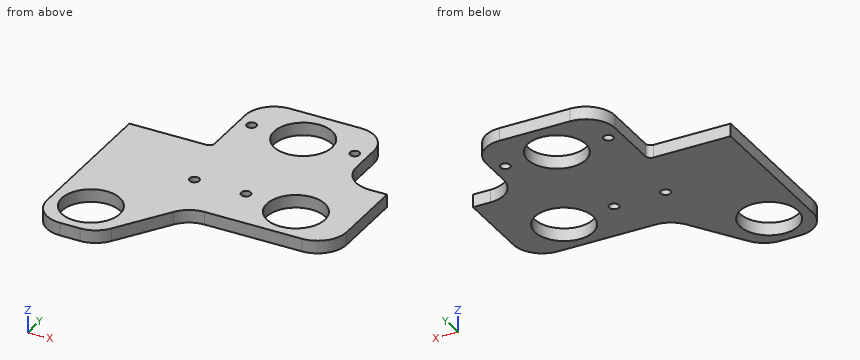
```python
from build123d import *

# Parameters (mm, degrees)
SKETCH1_R           = 14.3129
BOSS_EXTRUDE1_DEPTH = 6.35
FILLET1_R           = 14.2875
SKETCH2_W           = 63.5
SKETCH2_H           = 44.45
BOSS_EXTRUDE2_DEPTH = 6.35
FILLET2_R           = 14.2875
SKETCH3_R           = 14.3129
CUT_EXTRUDE1_DEPTH  = 110.433918417
SKETCH4_R           = 2.38125
SKETCH4_R_2         = 14.2875
CUT_EXTRUDE2_DEPTH  = 110.433918417
SKETCH5_R           = 2.38125
CUT_EXTRUDE3_DEPTH  = 110.433918417
FILLET3_R           = 2.54


with BuildPart() as part:
    # Sketch1 → Boss-Extrude1 (new body)
    with BuildSketch(Plane.XY):
        Polygon((-6.35, -6.35), (63.5, -6.35), (63.5, 44.45), (-63.5, 44.45), (-63.5, -44.45), (-31.75, -44.45), align=None)
        with Locations((-44.45, -25.4)):
            Circle(SKETCH1_R, mode=Mode.SUBTRACT)
        with Locations((35.871852568, 12.7)):
            Circle(SKETCH1_R, mode=Mode.SUBTRACT)
    extrude(amount=BOSS_EXTRUDE1_DEPTH)

    # Fillet1
    fillet1_edges = [part.edges().sort_by_distance(p)[0] for p in [
        (-31.75, -44.45, 3.175),
        (-63.5, -44.45, 3.175),
        (63.5, -6.35, 3.175),
        (-6.35, -6.35, 3.175),
    ]]
    fillet(fillet1_edges, radius=FILLET1_R)

    # Sketch2 → Boss-Extrude2 (add)
    with BuildSketch(Plane.XY.offset(6.35)):
        with Locations((8.89, 66.675)):
            Rectangle(SKETCH2_W, SKETCH2_H)
    extrude(amount=-BOSS_EXTRUDE2_DEPTH)

    # Fillet2
    fillet2_edges = [part.edges().sort_by_distance(p)[0] for p in [
        (-22.86, 88.9, 3.175),
        (40.64, 88.9, 3.175),
        (40.64, 44.45, 3.175),
    ]]
    fillet(fillet2_edges, radius=FILLET2_R)

    # Sketch3 → Cut-Extrude1 (cut, through all)
    with BuildSketch(Plane.XY.offset(6.35)):
        with Locations((9.062967637, 68.577618639)):
            Circle(SKETCH3_R)
    extrude(amount=-CUT_EXTRUDE1_DEPTH, mode=Mode.SUBTRACT)

    # Sketch4 → Cut-Extrude2 (cut, through all)
    with BuildSketch(Plane.XY.offset(6.35)):
        with Locations((-16.337032363, 68.577618639)):
            Circle(SKETCH4_R)
        with Locations((34.462967637, 68.577618639)):
            Circle(SKETCH4_R)
        with Locations((9.062967637, 68.577618639)):
            Circle(SKETCH4_R_2)
    extrude(amount=-CUT_EXTRUDE2_DEPTH, mode=Mode.SUBTRACT)

    # Sketch5 → Cut-Extrude3 (cut, through all)
    with BuildSketch(Plane.XY.offset(6.35)):
        with Locations((-15.875, 15.875)):
            Circle(SKETCH5_R)
        with Locations((9.525, 15.875)):
            Circle(SKETCH5_R)
    extrude(amount=-CUT_EXTRUDE3_DEPTH, mode=Mode.SUBTRACT)

    # Fillet3
    fillet3_edges = [part.edges().sort_by_distance(p)[0] for p in [
        (-22.86, 44.45, 3.175),
    ]]
    fillet(fillet3_edges, radius=FILLET3_R)


solid = part.part
```
Part model, mm, in its own coordinate system. Round coordinates to 2 decimals unless told otherwise and drop trailing zeros. Order: outer loops, then holes, each group sorted by start corner. A loop starts at its lowest first (then second) coordinate and runs counter-clockwise, first axis right, second up. Notation, with made-up numbers: M 37,46 L 72,46 A14 cw 72,70 Z; hole C -6.5,31.5 d11. An arc over 180 degrees is marked long. Answer in a Markdown table with one row per item. Add a question column.
Q1. Wall check: L1, parallel to Y at x = 9.5, z = 3; L2, parallel to Y at x = -15.5, z = 3.5 (3 decimals); L3, parallel to Y at x = 45, z = 5.25. Give the ranges that are in metal, low to high. Write a range as from..to.
Q2. Cut at A-A on x = -44.45. Give the cut face in (y, z), and give its area (3 significant figures).
Q3. Cut at B-B on y = -25.4. Give the cut face in (x, z), and give its area (3 significant figures).
Q4. Pin check, flat tips, straight feed: pin 1 (1.9 mm diameter, centred on y = 58.5, z = 4.5, fed in from -X); pin 2 (3 mm diameter, centred on y = 65, z = 1.5, fed in from +X); pin 3 (23 mm diameter, centred on x = 9.06, y = 68.58, fed in from -Z); pin 4 (1.9 mm diameter, centred on x = 35, z = 4.5, fed in from -Y). Stop position of each tip, or through.
Q5. Cut at C-C on z = 4. Give the number of separate pieces and of enclosed holes in the cut face, and give its area (3 significant figures).
Established:
| question | item | result |
|---|---|---|
| 1 | L1 | y = -6.35..13.49, 18.26..54.27, 82.88..88.9 |
| 1 | L2 | y = -20.075..13.523, 18.227..66.348, 70.807..87.108 |
| 1 | L3 | y = -6.35..1.68, 23.72..48.46 |
| 2 | outline | M -44.45,0 L -39.71,0 L -39.71,6.35 L -44.45,6.35 Z; M -11.09,0 L 44.45,0 L 44.45,6.35 L -11.09,6.35 Z |
| 2 | area | 383 mm2 |
| 3 | outline | M -63.5,0 L -58.76,0 L -58.76,6.35 L -63.5,6.35 Z; M -30.14,0 L -19.05,0 L -19.05,6.35 L -30.14,6.35 Z |
| 3 | area | 100 mm2 |
| 4 | pin 1 | stops at x = -22.86 |
| 4 | pin 2 | stops at x = 40.64 |
| 4 | pin 3 | passes through |
| 4 | pin 4 | stops at y = -6.35 |
| 5 | separate pieces | 1 |
| 5 | enclosed holes | 7 |
| 5 | area | 8,840 mm2 |
